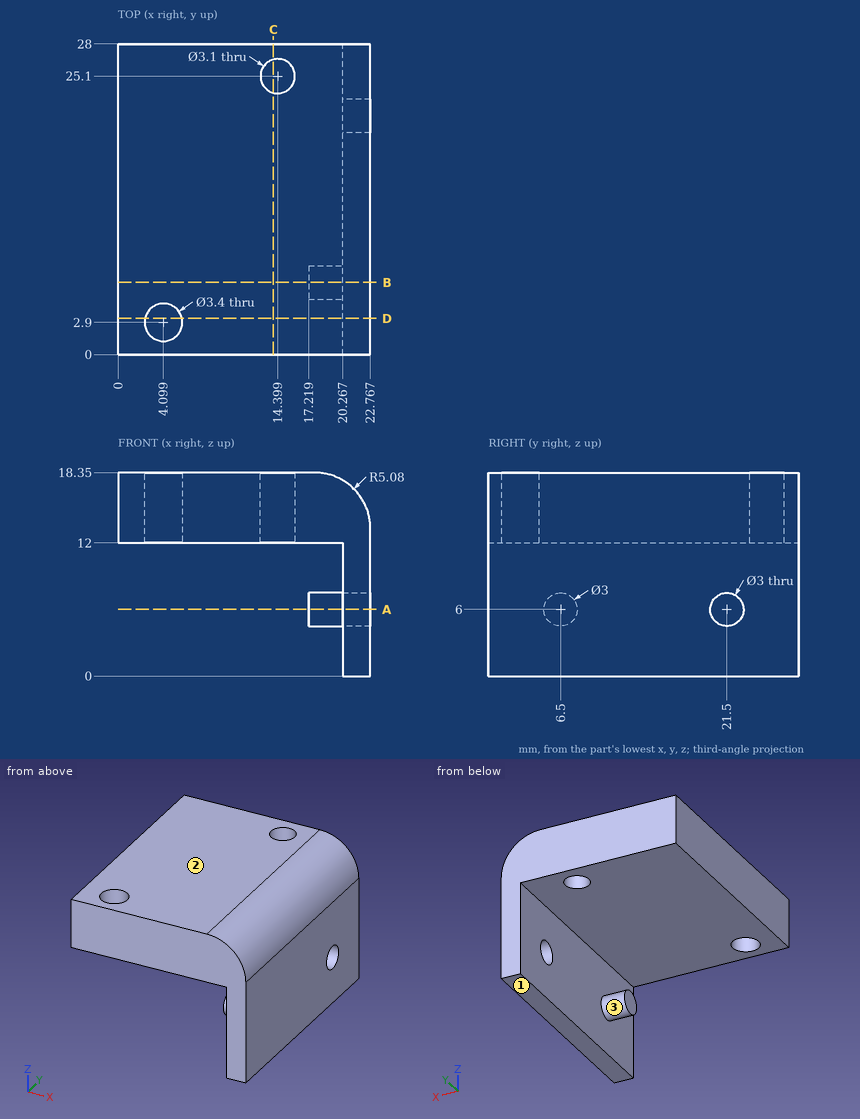
Could you check a few things on this drawing? It's one solid part, dimensions in mm from its lowest x, y, z. Round coordinates to 2 decimals unless told otherwise and drop trailing zeros. Order: outer loops, then holes, each group sorted by start corner. A loop starts at its lowest first (then second) coordinate and runs counter-clockwise, first axis right, second up. Notation, with made-up numbers: M 24.5,-33.5 L 62.5,-33.5 A32 ccw 62.5,-1.5 Z; hole C 47,50.5 d10. An arc over 180 degrees is marked long. One line per question, with ' | ' between items. Start each with the question number.
(1) Thinking about a two-plate mould opening in Z: for the marked faces 1, 2 and 3, which applies, +Z half, -Z half, draft (parallel to the pull), parting line (faces both ways), or undercut?
(2) For P1, Ø3.5, axis at y = 18, z = 7, coming from the -X side; P2, Ø8, axis at x = 7, z = 10.5, coming from the +Y side; P3, Ø6, axis at y = 8, z = 5.5, coming from the -X side; P4, Ø12, axis at x = 5.5, y = 20, coming from the -Z side, each with a flat end and sliding along its axis, tell me the tip position at first contact or that it passes through.
(3) Please list where these lines run through material, in increasing order: line 1 along Y through (x, z) = (22.05, 6); line 2 along X through (y, z) = (6.5, 9.5); line 3 along Z through (x, y) = (7, 10.5).
(4) Suppose I cut it at B-B on y = 6.5. List the corners of the cut face in (x, z) for me, then the cut area to 3 significant figures.
(5) Suppose I cut it at C-C on x = 14. List the corners of the cut face in (y, z) for me, then the cut area to 3 significant figures.
(6) Suppose I cut it at D-D on y = 3.25. List the corners of the cut face in (x, z) for me, then the cut area to 3 significant figures.
(7) Suppose I cut it at A-A on z = 6. List the corners of the cut face in (x, y) for me.
Geometry results:
1) face 1: -Z half | face 2: +Z half | face 3: undercut
2) P1: x = 20.27 | P2: y = 28 | P3: x = 17.22 | P4: z = 12
3) line 1: 0 to 20, 23 to 28 | line 2: 20.27 to 22.77 | line 3: 12 to 18.35
4) outline: M 0,12 L 20.27,12 L 20.27,7.5 L 17.22,7.5 L 17.22,4.5 L 20.27,4.5 L 20.27,0 L 22.77,0 L 22.77,13.27 A5.08 ccw 17.69,18.35 L 0,18.35 Z | area: 178 mm²
5) outline: M 0,12 L 23.6,12 L 23.6,18.35 L 0,18.35 Z; M 26.6,12 L 28,12 L 28,18.35 L 26.6,18.35 Z | area: 159 mm²
6) outline: M 0,12 L 2.44,12 L 2.44,18.35 L 0,18.35 Z; M 5.76,12 L 20.27,12 L 20.27,0 L 22.77,0 L 22.77,13.27 A5.08 ccw 17.69,18.35 L 5.76,18.35 Z | area: 148 mm²
7) outline: M 17.22,5 L 20.27,5 L 20.27,0 L 22.77,0 L 22.77,20 L 20.27,20 L 20.27,8 L 17.22,8 Z; M 20.27,23 L 22.77,23 L 22.77,28 L 20.27,28 Z
